For this review, take the finished solid that the model builds, in its own axes (mm). A direction names the side the tool comes from. Give positions to 0.01 mm unless a question says otherwise; leave off trailing zeros. Loops run counter-clockwise (first coordinate to the right, second up) from the corner with the lowest first, then second, coordinate; pieces in that order, holes last. Notation, with made-up numbers: (37.5, -0.75) -> (83.5, -0.75) arc R26 ccw to (83.5, 19.25) -> close; hole circle Ø10 at (-30.75, -12.75). An arc over 180 degrees is marked (long way). One line per question, with ' | ' between items. Start each with the question number.
(1) Consider section C-C (x = 21). Write out the cut boundary in (y, z), and give its area (3 significant figures).
(2) Consider section A-A (y = -16). Write out the cut boundary in (x, z) (3 decimals).
(3) Draft analysis for pull direction X (two halves, no side actions). For faces 1 (the cylindrical face through (-41.42, -10.96, 0.95)), 2 (the flat face through (-1, 1.27, 10)), 3 (the cylindrical face through (-7.559, 4.244, 5.796)), state which applies: +X half, -X half, draft (parallel to the pull), parting line (faces both ways), or undercut.
(4) Tool access review of faces 4 (the flat face through (-44, -22.225, 0)), 5 (the cylindrical face through (41.28, -10.96, 0.14)): name each direction out of +Z, -Z, +X, -X, +Y, -Y from which nothing blocks a thin tool from reaching the whole face with its end or side.
(5) Insertion check: P1, Ø8, axis at y = 8.5, z = 7, coming from the -X side; P2, Ø12, axis at x = 7.5, z = 8.5, coming from the +Y side; P3, Ø8, axis at x = -1, z = -5.5, coming from the -Y side. Each pin has a flat end and moves straight along its axis. Give the tip position at first contact, or say it passes through.
(6) Consider section B-B (x = 44.45). Write out the cut boundary in (y, z) (1 decimal).
(7) Wall thickness on probe 1 along Y at (x, z) = (23.5, -5.25); probe 2 along Z at (x, y) = (0, 3.5) (3 decimals); probe 3 along Z at (x, y) = (3, 10): over which ranges is each line inside the solid? List them lowest first.
from build123d import *

# Parameters (mm, degrees)
SKETCH1_W           = 98.425
SKETCH1_H           = 22.225
BOSS_EXTRUDE1_DEPTH = 1.27
SKETCH2_R           = 9.525
BOSS_EXTRUDE2_DEPTH = 14.2875
FILLET3_R           = 8.255
SKETCH3_R           = 3.175
BOSS_EXTRUDE3_DEPTH = 22.225


with BuildPart() as part:
    # Sketch1 → Boss-Extrude1 (new body)
    with BuildSketch(Plane(origin=(0, 0, 0), x_dir=(1, 0, 0), z_dir=(0, 1, 0))):
        Rectangle(SKETCH1_W, SKETCH1_H)
    extrude(amount=BOSS_EXTRUDE1_DEPTH)

    # Sketch2 → Boss-Extrude2 (add)
    with BuildSketch(Plane(origin=(0, 1.27, 0), x_dir=(1, 0, 0), z_dir=(0, 1, 0))):
        Circle(SKETCH2_R)
    extrude(amount=BOSS_EXTRUDE2_DEPTH)

    # Fillet3
    fillet3_edges = [part.edges().sort_by_distance(p)[0] for p in [
        (-9.525, 15.5575, 0),
    ]]
    fillet(fillet3_edges, radius=FILLET3_R)

    # Sketch3 → Boss-Extrude3 (add)
    with BuildSketch(Plane.XZ):
        with Locations((-44.45, 0)):
            Circle(SKETCH3_R)
        with Locations((44.45, 0)):
            Circle(SKETCH3_R)
    extrude(amount=BOSS_EXTRUDE3_DEPTH)


solid = part.part
A:
1) outline: (0, -11.11) -> (1.27, -11.11) -> (1.27, 11.11) -> (0, 11.11) -> close | area: 28.2 mm^2
2) outline: circle Ø6.35 at (-44.45, 0); circle Ø6.35 at (44.45, 0)
3) face 1: undercut | face 2: draft | face 3: parting line
4) face 4: +Z, -Z, +X, -X, -Y | face 5: -Y
5) P1: stops at x = -9 | P2: stops at y = 14.49 | P3: stops at y = 0
6) outline: (-22.2, -3.2) -> (0, -3.2) -> (0, -11.1) -> (1.3, -11.1) -> (1.3, 11.1) -> (0, 11.1) -> (0, 3.2) -> (-22.2, 3.2) -> close
7) probe 1: y = 0 to 1.27 | probe 2: z = -9.525 to 9.525 | probe 3: z = -8.56 to 8.56
